```python
from build123d import *

# Parameters (mm, degrees)
BOSS_EXTRUDE1_DEPTH = 2.7
FILLET1_R           = 0.5


with BuildPart() as part:
    # Sketch1 → Boss-Extrude1 (new body)
    with BuildSketch(Plane.XY):
        with BuildLine():
            Line((-3.25, 1.75), (3.25, 1.75))
            ThreePointArc((3.25, 1.75), (5, 0), (3.25, -1.75))
            Line((3.25, -1.75), (-3.25, -1.75))
            ThreePointArc((-3.25, -1.75), (-5, 0), (-3.25, 1.75))
        make_face()
    extrude(amount=BOSS_EXTRUDE1_DEPTH)

    # Fillet1
    fillet1_edges = [part.edges().sort_by_distance(p)[0] for p in [
        (5, 0, 2.7),
        (0, 1.75, 2.7),
        (-5, 0, 2.7),
        (0, -1.75, 2.7),
    ]]
    fillet(fillet1_edges, radius=FILLET1_R)


solid = part.part
```
CAD build for the part. Positions are in the model's coordinates, mm. Coordinates: 2 decimals unless noted, no trailing zeros. Order: outer loops, then holes, each group sorted by start corner. A loop starts at its lowest first (then second) coordinate and runs counter-clockwise, first axis right, second up.
(1) Drill centre lines: L1, parallel to X at y = -1.5, z = 1.6; L2, parallel to X at y = -1.15, z = 0.75; L3, parallel to Y at x = 2.25, z = 2.4. Where is each one in solid material? Low to high.
Solution:
L1: x = -4.15 to 4.15
L2: x = -4.57 to 4.57
L3: y = -1.71 to 1.71
(2) Mould opens along Z. For faces 1 (the face through (0, 0, 2.7)), 2 (the face through (0, -1.75, 1)), 3 (the face through (0, 0, 0)) say: released by +Z, released by -Z, zero draft, split by the parting line, or undercut.
Solution:
face 1: released by +Z
face 2: zero draft
face 3: released by -Z
(3) Saw through at A-A, the plane z = 1.8. Write the cut outline in (x, y).
Solution:
outline: (-3.25, -1.75) - (3.25, -1.75) arc R1.75 ccw to (3.25, 1.75) - (-3.25, 1.75) arc R1.75 ccw to start
(4) Saw through at B-B, the plane z = 2.5. Write the cut outline in (x, y).
Solution:
outline: (-3.25, -1.65) - (3.25, -1.65) arc R1.65 ccw to (3.25, 1.65) - (-3.25, 1.65) arc R1.65 ccw to start
